Geometry: see drawing. Coordinates: mm, zero at the bounding-box minimum. A direction names the side the tool comes from. Give positions to 0.01 mm unless a question says otherwise; leave off trailing zeros. Write each loop counter-clockwise with the first axis right and the second up, starting at its lowest first coordinate (ties: lowest second). Pieces come first, ordered by that corner, then holes. Notation, with made-up numbers: (-9.75, 12) -> (42.25, 12) arc R17 ccw to (42.25, 19) -> close; hole circle Ø11 at (42.25, 59). An arc over 180 degrees is marked (long way). Use CSV: the item, a comma, the result in double quotes. Start each with the question number.
1) Section C-C (z = 3.5). Output: boundary loops of the cut face in (x, y).
2) Section A-A (y = 4). Output: boundary loops of the cut face in (x, z), plus the area to 3 significant figures.
3) Material intervals for line 1 (Y direction, x = 4, z = 0.35); line 2 (Y direction, x = 6.75, z = 12.75); line 3 (Z direction, x = 0.75, y = 3), sorted ascending. Write a range as [from, to].
4) Contact query for flat-ended pins moving along their axis: P1, Ø1.5, axis at x = 3.5, y = 9, coming from the +Z side; P2, Ø1.5, axis at x = 5.5, z = 8.5, coming from the +Y side; P3, Ø0.9, axis at y = 10, z = 2.5, coming from the +X side; P4, Ø5, axis at y = 9.5, z = 10.5, coming from the +X side. Output: stop coordinate, or through.
5) Set-up query: the marked faces 4, 5 and 6. Return all of +Z, -Z, +X, -X, +Y, -Y with unobstructed straight access to the full face (end or side cutting, diameter ignored); none if empty.
6) Draft query along X for the marked faces 1, 2 and 3. Return one class per face: pulls with the +X half, pulls with the -X half, needs draft (parallel to the pull), parting line crosses it, or undercut.
7) Section B-B (x = 4). Output: boundary loops of the cut face in (y, z).
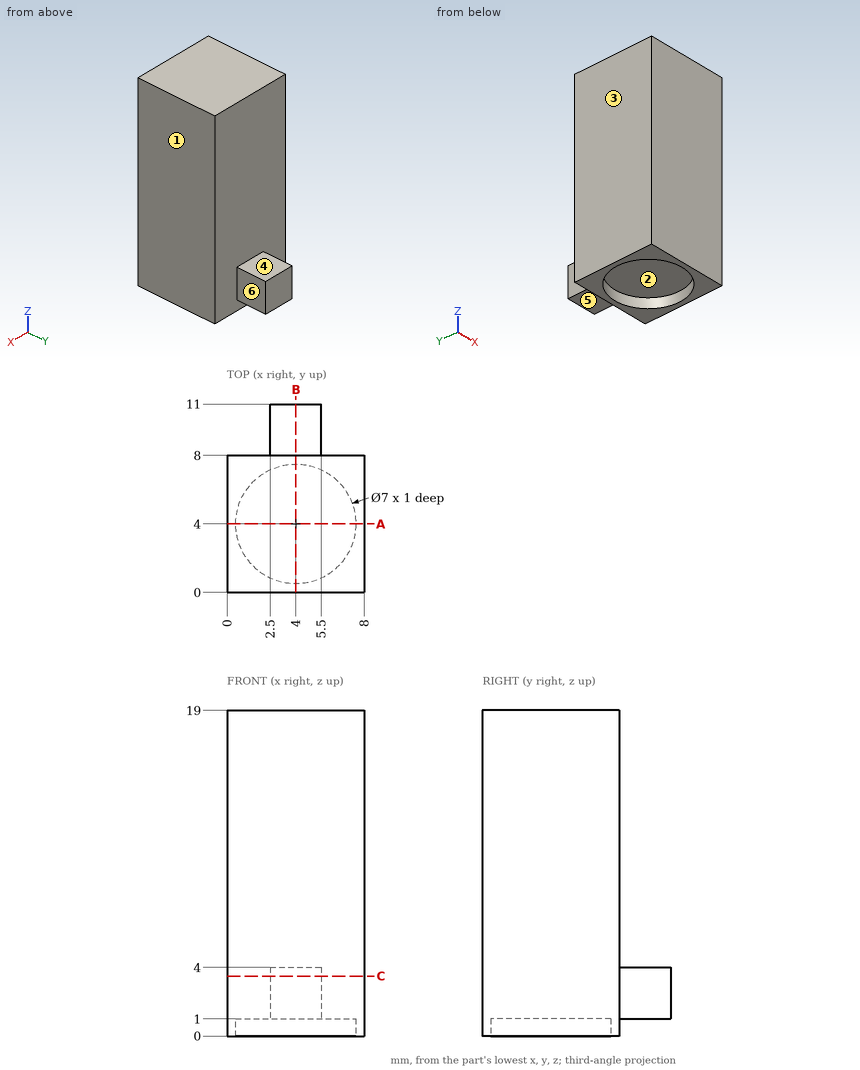
Answers follow:
1,outline,"(0, 0) -> (8, 0) -> (8, 8) -> (5.5, 8) -> (5.5, 11) -> (2.5, 11) -> (2.5, 8) -> (0, 8) -> close"
2,outline,"(0, 0) -> (0.5, 0) -> (0.5, 1) -> (7.5, 1) -> (7.5, 0) -> (8, 0) -> (8, 19) -> (0, 19) -> close"
2,area,"145 mm^2"
3,line 1,"y = [0, 0.5], [7.5, 8]"
3,line 2,"y = [0, 8]"
3,line 3,"z = [1, 19]"
4,P1,"stops at z = 4"
4,P2,"stops at y = 8"
4,P3,"stops at x = 5.5"
4,P4,"stops at x = 8"
5,face 4,"+Z, +X, -X, +Y"
5,face 5,"-Z, +X, -X, +Y"
5,face 6,"+Z, -Z, +X, +Y"
6,face 1,"pulls with the +X half"
6,face 2,"undercut"
6,face 3,"pulls with the -X half"
7,outline,"(0, 0) -> (0.5, 0) -> (0.5, 1) -> (7.5, 1) -> (7.5, 0) -> (8, 0) -> (8, 1) -> (11, 1) -> (11, 4) -> (8, 4) -> (8, 19) -> (0, 19) -> close"
